```python
from build123d import *

# Parameters (mm, degrees)
F1_DEPTH = 20
F3_DEPTH = 50
F5_DEPTH = 20


with BuildPart() as f1:
    # F0 (on Top) → F1 (new body)
    with BuildSketch(Plane.XY):
        Polygon((-19.75, -17.7500005811), (-19.75, -19.75), (-13.75, -19.75), (19.75, 13.75), (19.75, 19.75), (17.7500005811, 19.75), (17.7500005811, 14.578426884), (-14.578426884, -17.7500005811), align=None)
    extrude(amount=F1_DEPTH)

    # F2 (on face) → F3 (join)
    with BuildSketch(Plane.XY.offset(20)):
        Polygon((-19.75, -19.75), (-13.75, -19.75), (19.75, 13.75), (19.75, 19.75), (11.25, 19.75), (11.25, 28.25), (7.75, 24.75), (7.75, 22.75), (9.25, 22.75), (9.25, 19.7500005811), (7.75, 19.7500005811), (7.75, 17.7500005811), (14.3357871391, 11.164213442), (-11.164213442, -14.3357871391), (-17.7500005811, -7.75), (-19.7500005811, -7.75), (-19.7500005811, -9.25), (-22.75, -9.25), (-22.75, -7.75), (-24.75, -7.75), (-28.25, -11.25), (-19.75, -11.25), align=None)
        Polygon((-14.578426884, -17.7500005811), (-17.7500005811, -17.7500005811), (-17.7500005811, -10.5784263029), (-12.5784265935, -15.7500002906), align=None, mode=Mode.SUBTRACT)
        Polygon((10.5784263029, 17.7500005811), (17.7500005811, 17.7500005811), (17.7500005811, 14.578426884), (15.7500002906, 12.5784265935), align=None, mode=Mode.SUBTRACT)
    extrude(amount=F3_DEPTH)

    # F5 (cut, through all): a face of the model
    f5_faces = [f1.faces().sort_by_distance(p)[0] for p in [
        (2.0288816122, -2.0288816122, 0),
    ]]
    extrude(f5_faces, amount=-F5_DEPTH, mode=Mode.SUBTRACT)


solid = f1.part
```
Design review of the part built by this model. Coordinates are the model's own, in mm. A direction names the side the tool comes from. Round coordinates to 2 decimals unless told otherwise and drop trailing zeros. Order: outer loops, then holes, each group sorted by start corner. A loop starts at its lowest first (then second) coordinate and runs counter-clockwise, first axis right, second up. Notation, with made-up numbers: M 47.5,51.5 L 93.5,51.5 A11 cw 93.5,66.5 Z; hole C -39.75,56 d8. An arc over 180 degrees is marked long. Put each result on its own line as item: value.
Q1. Insertion check: pin 1 Ø2 at (x, z) = (-24, 57) entering from +Y; pin 2 Ø1.6 at (y, z) = (-8.5, 40.5) entering from -X; pin 3 Ø2 at (y, z) = (7, 56) entering from +X. Each pin has a flat end and moves straight along its axis. Give the tip position at first contact, or say it passes through.
Reported:
pin 1: y = -7.75
pin 2: x = -26.3
pin 3: x = 14
Q2. Consider section A-A (z = 39). State how many separate pieces and enclosed holes the cut face has, and give its area (3 significant figures).
Reported:
separate pieces: 1
enclosed holes: 2
area: 227 mm²
Q3. To check wall thickness, follow line 1 (Y direction, x = 13, z = 67); line 2 (X direction, y = -14, z = 32.5); line 3 (Y direction, x = -19, z = 37.5). State the ranges of each line that lie inside material, in increasing order.
Reported:
line 1: 7 to 9.83, 12.5 to 15.33, 17.75 to 19.75
line 2: -19.75 to -17.75, -14.33 to -11.5, -10.83 to -8
line 3: -19.75 to -7.75
Q4. Consider section B-B (y = -8.5). State the section outline as (x, z) points, and give its area (3 significant figures).
Reported:
outline: M -25.5,20 L -22.75,20 L -22.75,70 L -25.5,70 Z; M -19.75,20 L -17,20 L -17,70 L -19.75,70 Z; M -5.33,20 L -2.5,20 L -2.5,70 L -5.33,70 Z
area: 416 mm²
Q5. Machinability: for faces 1 (the face through (11, 14.5, 44.6)), 2 (the face through (-24, -11.25, 45)), 3 (the face through (-24, -7.75, 45)), which of the approach directions +Z, -Z, +X, -X, +Y, -Y give a long, thin tool a straight path to every point of the face, cutting with its end or side? Answer none if there is none.
Reported:
face 1: +Z, -Z, -X
face 2: +Z, -Z, -X, -Y
face 3: +Z, -Z, -X, +Y
Q6. Draft analysis for pull direction Y (two halves, no side actions). For faces 4 (the face through (-13.564, -16.736, 44.65)), 5 (the face through (1, -3, 70)), 6 (the face through (-17, -19.75, 45)), state which applies: released by +Y, released by -Y, zero draft, split by the parting line, or undercut.
Reported:
face 4: undercut
face 5: zero draft
face 6: released by -Y
Q7. Consider section D-D (y = 17). State the section outline as (x, z) points, and give its area (3 significant figures).
Reported:
outline: M 8.5,20 L 11.33,20 L 11.33,70 L 8.5,70 Z; M 17.75,20 L 19.75,20 L 19.75,70 L 17.75,70 Z
area: 241 mm²
Q8. Consider section C-C (x = 16.5). State the section outline as (y, z) points.
Reported:
outline: M 10.5,20 L 13.33,20 L 13.33,70 L 10.5,70 Z; M 17.75,20 L 19.75,20 L 19.75,70 L 17.75,70 Z
